from build123d import *

# Parameters (mm, degrees)
SKETCH1_W            = 44.45
SKETCH1_H            = 55.05
BOSS_EXTRUDE1_DEPTH  = 6.35
SKETCH2_W            = 2.7
SKETCH2_H            = 19.05
CUT_EXTRUDE1_DEPTH   = 53.666408886
M6_CLEARANCE_HOLE1_D = 6.6


with BuildPart() as part:
    # Sketch1 → Boss-Extrude1 (new, symmetric)
    with BuildSketch(Plane(origin=(0, 0, 0), x_dir=(0, 0, -1), z_dir=(1, 0, 0))):
        Rectangle(SKETCH1_W, SKETCH1_H)
    extrude(amount=BOSS_EXTRUDE1_DEPTH, both=True)

    # Sketch2 → Cut-Extrude1 (cut, through all)
    with BuildSketch(Plane(origin=(0, 0, -22.225), x_dir=(-1, 0, 0), z_dir=(0, 0, -1))):
        with Locations((-5, -18)):
            Rectangle(SKETCH2_W, SKETCH2_H)
    extrude(amount=-CUT_EXTRUDE1_DEPTH, mode=Mode.SUBTRACT)

    # M6 Clearance Hole1 (through all)
    with Locations(Plane(origin=(0, -27.525, 0), x_dir=(-1, 0, 0), z_dir=(0, -1, 0))):
        with Locations((1.35, 15), (1.35, -15)):
            Hole(M6_CLEARANCE_HOLE1_D / 2)


solid = part.part
Part model, mm, in its own coordinate system. A direction names the side the tool comes from. Coordinates: 2 decimals unless noted, no trailing zeros. Order: outer loops, then holes, each group sorted by start corner. A loop starts at its lowest first (then second) coordinate and runs counter-clockwise, first axis right, second up. Notation, with made-up numbers: M 60.5,-14 L 114.5,-14 A30 cw 114.5,14 Z; hole C -24.75,59 d8. An arc over 180 degrees is marked long. One line per question, with ' | ' between items.
Q1. Slice it at C-C (z = 15). Give the cut face in (x, y) (3 decimals), and give its area (3 significant figures).
A:
outline: M -6.35,-27.525 L -4.65,-27.525 L -4.65,27.525 L -6.35,27.525 Z; M 1.95,-27.525 L 3.65,-27.525 L 3.65,-8.475 L 6.35,-8.475 L 6.35,27.525 L 1.95,27.525 Z | area: 284 mm^2
Q2. Drill centre lines: line 1 (Z direction, x = -1.35, y = -4) (3 decimals); line 2 (X direction, y = 14, z = 15); line 3 (Z direction, x = -2.25, y = 12) (3 decimals). Where is each one in solid material? Low to high.
A:
line 1: z = -22.225 to -18.3, -11.7 to 11.7, 18.3 to 22.225 | line 2: x = -6.35 to -4.65, 1.95 to 6.35 | line 3: z = -22.225 to -18.175, -11.825 to 11.825, 18.175 to 22.225
Q3. Slice it at D-D (z = -1). Give the cut face in (x, y) (3 decimals), and give its area (3 significant figures).
A:
outline: M -6.35,-27.525 L 3.65,-27.525 L 3.65,-8.475 L 6.35,-8.475 L 6.35,27.525 L -6.35,27.525 Z | area: 648 mm^2
Q4. Slice it at B-B (y = -13.5). Give the cut face in (x, z) (3 decimals), and give its area (3 significant figures).
A:
outline: M -6.35,-22.225 L 3.65,-22.225 L 3.65,22.225 L -6.35,22.225 Z; hole C -1.35,-15 d6.6; hole C -1.35,15 d6.6 | area: 376 mm^2
Q5. Pin check, flat tips, straight feed: P1, Ø0.8, axis at x = 5, z = 0.5, coming from the -Y side (3 decimals); P2, Ø15, axis at y = -20, z = 4, coming from the +X side. Stop position of each tip, or through.
A:
P1: stops at y = -8.475 | P2: stops at x = 3.65
Q6. Two-plate mould, pull along X, no slides. Class faces 3 (the face through (0, 27.525, 0)), 4 (the face through (3.65, -18, 0)), 5 (the face through (-3.969, 0.385, 17.008)): +X half, -X half, draft (parallel to the pull), parting line (faces both ways), or undercut.
A:
face 3: draft | face 4: +X half | face 5: undercut
Q7. Slice it at A-A (x = -1.35). Give the cut face in (y, z) (3 decimals).
A:
outline: M -27.525,-22.225 L 27.525,-22.225 L 27.525,-18.3 L -27.525,-18.3 Z; M -27.525,-11.7 L 27.525,-11.7 L 27.525,11.7 L -27.525,11.7 Z; M -27.525,18.3 L 27.525,18.3 L 27.525,22.225 L -27.525,22.225 Z
Q8. 3-axis set-ups, long thin cutter, end or side, ignore diameter. For faces 1 (the face through (0, 0, -22.225)), 2 (the face through (5, -8.475, 0)): which of +Z, -Z, +X, -X, +Y, -Y reach the whole face in a straight line?
A:
face 1: -Z, +X, -X, +Y, -Y | face 2: +Z, -Z, +X, -Y
